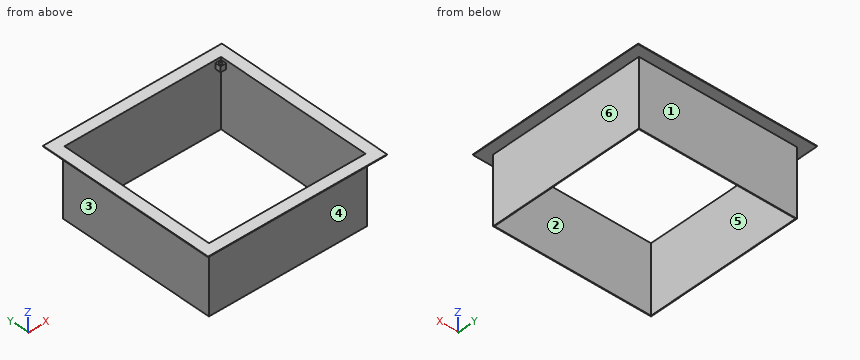
from build123d import *

# Parameters (mm, degrees)
F0_W     = 812.8
F0_H     = 812.8
F0_W_2   = 711.2
F0_H_2   = 711.2
F1_DEPTH = 3.175
F2_W     = 717.55
F2_H     = 717.55
F2_W_2   = 711.2
F2_H_2   = 711.2
F3_DEPTH = 304.8
F4_W     = 25.4
F4_H     = 25.4
F5_DEPTH = 25.4
F6_R     = 6.35
F7_DEPTH = 25.4


with BuildPart() as f1:
    # F0 (on Top) → F1 (new body)
    with BuildSketch(Plane.XY):
        Rectangle(F0_W, F0_H)
        Rectangle(F0_W_2, F0_H_2, mode=Mode.SUBTRACT)
    extrude(amount=F1_DEPTH)

    # F2 (on face) → F3 (join)
    with BuildSketch(Plane(origin=(0, 0, 0), x_dir=(1, 0, 0), z_dir=(0, 0, -1))):
        Rectangle(F2_W, F2_H)
        Rectangle(F2_W_2, F2_H_2, mode=Mode.SUBTRACT)
    extrude(amount=F3_DEPTH)

    # F4 (on face) → F5 (join)
    with BuildSketch(Plane.XZ.offset(-355.6)):
        with Locations((342.9, -22.225)):
            Rectangle(F4_W, F4_H)
    extrude(amount=F5_DEPTH)

    # F6 (on face) → F7 (cut, through all)
    with BuildSketch(Plane.XY.offset(-9.525)):
        with Locations((342.9, 342.9)):
            Circle(F6_R)
    extrude(amount=-F7_DEPTH, mode=Mode.SUBTRACT)


solid = f1.part
Check sheet for the modelled part. Datum: model origin and axes. Units: mm. Face numbers are marked on the shaded views. A direction names the side the tool comes from. Round coordinates to 2 decimals unless told otherwise and drop trailing zeros. Order: outer loops, then holes, each group sorted by start corner. A loop starts at its lowest first (then second) coordinate and runs counter-clockwise, first axis right, second up.
(1) Go/stop test with flat-tipped pins: P1, Ø8, axis at x = -266.5, z = -38, coming from the +Y side (3 decimals); P2, Ø3, axis at y = -302, z = -129, coming from the -X side (3 decimals); P3, Ø12.5, axis at x = 337.5, z = -18.5, coming from the -Y side (3 decimals). Record where each tip stops, or that it passes through.
(2) Cross-section at C-C, the plane z = -93. Enter the section's corners in (x, y) (3 decimals), and give its area (3 significant figures).
(3) Access from +Z, -Z, +X, -X, +Y, -Y to the whole of each face (thin tool, end or side, straight path). Record for the marked faces 4, 5 and 6.
(4) Draft check along X on the marked faces 1, 2 and 3. Enter one of: pulls with the +X half, pulls with the -X half, needs draft (parallel to the pull), parting line crosses it, or undercut.
(5) Scan lines: probe 1 along X at (y, z) = (342.9, -17.5) (3 decimals); probe 2 along Y at (x, z) = (342, -22) (3 decimals); probe 3 along Y at (x, z) = (212, -178.5) (3 decimals). Record each from-to range of solid material in increasing order.
(6) Cross-section at A-A, the plane x = -270. Enter the section's corners in (y, z) (3 decimals), and give its area (3 significant figures).
Check sheet entries:
1. P1: stops at y = 358.775
1. P2: stops at x = -358.775
1. P3: stops at y = -358.775
2. outline: (-358.775, -358.775) - (358.775, -358.775) - (358.775, 358.775) - (-358.775, 358.775) - close; hole (-355.6, -355.6) - (355.6, -355.6) - (355.6, 355.6) - (-355.6, 355.6) - close
2. area: 9,070 mm2
3. face 4: -Z, +X, -X, -Y
3. face 5: +Z, -Z
3. face 6: -Z, +X, +Y, -Y
4. face 1: needs draft
4. face 2: undercut
4. face 3: pulls with the -X half
5. probe 1: x = -358.775 to -355.6, 330.2 to 336.55, 349.25 to 358.775
5. probe 2: y = -358.775 to -355.6, 330.2 to 336.614, 349.186 to 358.775
5. probe 3: y = -358.775 to -355.6, 355.6 to 358.775
6. outline: (-406.4, 0) - (-358.775, 0) - (-358.775, -304.8) - (-355.6, -304.8) - (-355.6, 3.175) - (-406.4, 3.175) - close; (355.6, -304.8) - (358.775, -304.8) - (358.775, 0) - (406.4, 0) - (406.4, 3.175) - (355.6, 3.175) - close
6. area: 2,260 mm2
